Here's how the part is built. I have some questions about the finished solid (model axes, mm). Face numbers are marked on the shaded views. A direction names the side the tool comes from. Coordinates: 2 decimals unless noted, no trailing zeros. Write each loop counter-clockwise with the first axis right and the second up, starting at its lowest first coordinate (ties: lowest second). Pieces come first, ordered by that corner, then holes.
Item 1: Please list where these lines run through material, in increasing order: line 1 (Z direction, x = -27.5, y = -11.5); line 2 (Y direction, x = -25, z = 15); line 3 (Y direction, x = 13.5, z = -8).
Item 2: If we mould it in two halves opening along X, with no side actions, what happens to the marked faces 1, 2 and 3? For each: pulls with the +X half, pulls with the -X half, needs draft (parallel to the pull), parting line crosses it, or undercut.
Item 3: I'm going to push flat-ended pins straight in: P1, Ø4, axis at y = -25.5, z = -8.5, coming from the +X side; P2, Ø10, axis at y = -5, z = 7.5, coming from the -X side; P3, Ø12, axis at y = -21.5, z = 13, coming from the +X side. Where does each tip first touch, or does it pass through?
Item 4: I want a section at D-D (z = 2). Please give me the cut outline in (x, y), and give its area (3 significant figures).
Item 5: I want a section at C-C (x = 17.5). Please give me the cut outline in (y, z), and give its area (3 significant figures).
Item 6: For the marked faces 4, 5, 6 and 7, which set-ups out of +Z, -Z, +X, -X, +Y, -Y let a thin tool reach every point of the face, with its end or its side?
Item 7: I want a section at B-B (y = -11). Please give me the cut outline in (x, z), and give its area (3 significant figures).
Item 8: I want a section at A-A (z = -7.5). Please give me the cut outline in (x, y), and give its area (3 significant figures).
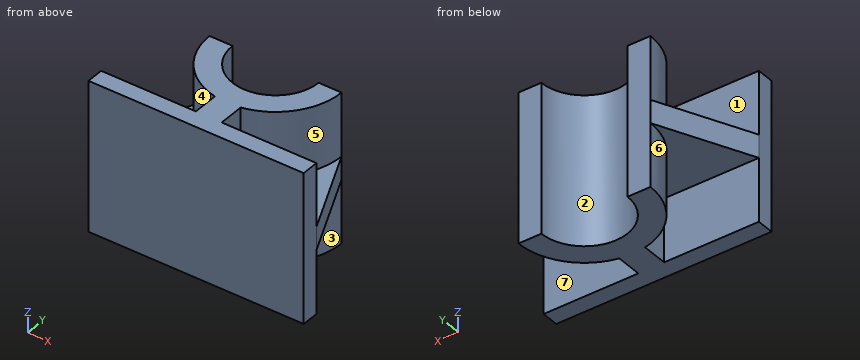
from build123d import *

# Parameters (mm, degrees)
BOSS_EXTRUDE1_DEPTH = 26
RIB1_REACH          = 61.099
SKETCH2_WALL_W      = 154.925032954
SKETCH2_WALL_H      = 8


with BuildPart() as part:
    # Sketch1 → Boss-Extrude1 (new, symmetric)
    with BuildSketch(Plane.XY):
        with BuildLine():
            Line((-37.5, -37.555487137), (0, -37.555487137))
            Line((0, -37.555487137), (0, -15))
            ThreePointArc((0, -15), (-10.606601718, -10.606601718), (-15, 0))
            Line((-15, 0), (-23, 0))
            ThreePointArc((-23, 0), (-17.783419244, -14.585952146), (-4.5, -22.555487137))
            Line((-4.5, -22.555487137), (-4.5, -31.555487137))
            Line((-4.5, -31.555487137), (-37.5, -31.555487137))
            Line((-37.5, -31.555487137), (-37.5, -37.555487137))
        make_face()
        with BuildLine():
            Line((0, -37.555487137), (37.5, -37.555487137))
            Line((37.5, -37.555487137), (37.5, -31.555487137))
            Line((37.5, -31.555487137), (4.5, -31.555487137))
            Line((4.5, -31.555487137), (4.5, -22.555487137))
            ThreePointArc((4.5, -22.555487137), (17.783419244, -14.585952146), (23, 0))
            Line((23, 0), (15, 0))
            ThreePointArc((15, 0), (10.606601718, -10.606601718), (0, -15))
            Line((0, -15), (0, -37.555487137))
        make_face()
    extrude(amount=BOSS_EXTRUDE1_DEPTH, both=True)

    # Sketch2 wall → Rib1 (add, up to next)
    with BuildSketch(Plane(origin=(30.25, -15.777743569, 0), x_dir=(0.417536618888, -0.908660097004, 0), z_dir=(0.908660097004, 0.417536618888, 0)), mode=Mode.PRIVATE) as rib1_sk1:
        Rectangle(SKETCH2_WALL_W, SKETCH2_WALL_H)
    rib1_tool1 = extrude(rib1_sk1.sketch, amount=-RIB1_REACH, mode=Mode.PRIVATE) - part.part
    rib1 = rib1_tool1.solids().sort_by_distance((30.25, -15.777743569, 0))[0]
    add(rib1)

    # Mirror1: Rib1 across plane
    add(rib1.mirror(Plane(origin=(0, 0, 0), x_dir=(0, 0, 1), z_dir=(1, 0, 0))))


solid = part.part
Answer:
1. line 1: z = -4 to 4
1. line 2: y = -37.56 to -31.56
1. line 3: y = -37.56 to -31.56, -18.62 to -6.54
2. face 1: needs draft
2. face 2: undercut
2. face 3: pulls with the +X half
3. P1: stops at x = 4.5
3. P2: stops at x = -26.94
3. P3: stops at x = 16.99
4. outline: (-37.5, -37.56) - (37.5, -37.56) - (37.5, -31.56) - (23, 0) - (15, 0) arc R15 cw to (-15, 0) - (-23, 0) - (-37.5, -31.56) - close
4. area: 2,010 mm2
5. outline: (-37.56, -26) - (-31.56, -26) - (-31.56, -4) - (-14.92, -4) - (-14.92, -26) - (0, -26) - (0, 26) - (-14.92, 26) - (-14.92, 4) - (-31.56, 4) - (-31.56, 26) - (-37.56, 26) - close
5. area: 1,220 mm2
6. face 4: +Z, -X
6. face 5: +Z, +X
6. face 6: -Z, -X
6. face 7: -Z, +X
7. outline: (-28.05, -4) - (-20.2, -4) - (-20.2, -26) - (-10.2, -26) - (-10.2, 26) - (-20.2, 26) - (-20.2, 4) - (-28.05, 4) - close; (10.2, -26) - (20.2, -26) - (20.2, -4) - (28.05, -4) - (28.05, 4) - (20.2, 4) - (20.2, 26) - (10.2, 26) - close
7. area: 1,170 mm2
8. outline: (-37.5, -37.56) - (37.5, -37.56) - (37.5, -31.56) - (4.5, -31.56) - (4.5, -22.56) arc R23 ccw to (23, 0) - (15, 0) arc R15 cw to (-15, 0) - (-23, 0) arc R23 ccw to (-4.5, -22.56) - (-4.5, -31.56) - (-37.5, -31.56) - close
8. area: 1,010 mm2
